Geometry: final body of the model. Coordinates: model frame, mm. A direction names the side the tool comes from. Coordinates: 2 decimals unless noted, no trailing zeros. Order: outer loops, then holes, each group sorted by start corner. A loop starts at its lowest first (then second) coordinate and runs counter-clockwise, first axis right, second up. Notation, with made-up numbers: (-30, 22.25) -> (20, 22.25) arc R9 ccw to (20, 27.25) -> close; hole circle Ø8 at (88, -23.5). An arc over 180 degrees is marked (long way). Answer in a Markdown table with one row per item. Add a question column.
1) Contact query for flat-ended pins moving along their axis: P1, Ø0.8, axis at y = 6.5, z = 29.5, coming from the +X side; P2, Ø0.6, axis at x = 14.5, z = 29.5, coming from the -Y side; P3, Ø1, axis at x = 14, z = 4.5, coming from the +Y side. Output: stop coordinate, or through.
2) Section query A-A on y = 9.5. Return the cut outline in (x, z), then the cut area to 4 significant figures.
3) Ray query, line 1 (Y direction, x = 4.5, z = 3); line 2 (X direction, y = 2.5, z = 20.5); line 3 (Z direction, x = 10.25, y = 13). Return the intervals inside material, ascending. Write a range as from..to.
4) Set-up query: faces 5 (the face through (14, 8, 1.5)), 6 (the face through (-0.5, 8, 29)), 7 (the face through (7, 16, 15)). Return all of +Z, -Z, +X, -X, +Y, -Y with unobstructed straight access to the full face (end or side cutting, diameter ignored); none if empty.
5) Pull-direction query (Y, two-part tool) for faces 1 (the face through (7, -1.3, 13)), 2 (the face through (7, 0, 15)), 3 (the face through (7, 27, -4)), 4 (the face through (14.5, 8, 7)); classes: +Y half, -Y half, draft (parallel to the pull), parting line (faces both ways), or undercut.
6) Section query C-C on x = 5. Return the cut outline in (y, z).
7) Section query B-B on z = -1.5. Return the cut outline in (x, y), then the cut area to 3 significant figures.
8) Section query D-D on z = 10. Return the cut outline in (x, y).
Autodesk Inventor part; units mm, degrees
ref_plane "Work Plane1" through (6.6, -1.3, -3) normal (1, 0, 0) x (0, 0, -1)
ref_plane "YZ Plane" through (0, 0, 0) normal (1, 0, 0) x (0, 1, 0)
ref_plane "XZ Plane" through (0, 0, 0) normal (0, 1, 0) x (-1, 0, 0)
sketch "Sketch1" plane through (0, 0, 0) normal (0, 0, 1) x (1, 0, 0)
  point P0 (0, 0)
sketch "Sketch2" plane through (0, 0, 0) normal (0, 0, 1) x (1, 0, 0)
  line L0 (0, 0) -> (13.2, 0)
  line L1 (13.2, 0) -> (13.2, 16)
  line L2 (13.2, 16) -> (0, 16)
  line L3 (0, 16) -> (0, 0)
  line L4 (14.5, 17.3) -> (14.5, -1.3)
  line L5 (14.5, -1.3) -> (-1.3, -1.3)
  line L6 (-1.3, -1.3) -> (-1.3, 17.3)
  line L7 (-1.3, 17.3) -> (14.5, 17.3)
  dimension "d0" = 13.2
  dimension "d1" = 16
  dimension "d2" = 1.3
extrude "Extrusion1" add sketch "Sketch2" along normal blind 30
sketch "Sketch3" plane through (0, 0, 0) normal (0, 0, -1) x (-1, 0, 0)
  line L0 (-14.5, -1.3) -> (-14.5, 17.3)
  line L1 (1.3, 17.3) -> (1.3, -1.3)
  line L2 (-14.5, 17.3) -> (1.3, 17.3)
  line L3 (1.3, -1.3) -> (-14.5, -1.3)
  line L4 (1.3, 17.3) -> (-14.5, 17.3)
  line L5 (-14.5, 17.3) -> (-14.5, 25.3)
  line L6 (-14.5, 25.3) -> (1.3, 25.3)
  line L7 (1.3, 25.3) -> (1.3, 17.3)
  line L8 (1.3, -1.3) -> (-14.5, -1.3)
  line L9 (-14.5, -1.3) -> (-14.5, -9.3)
  line L10 (-14.5, -9.3) -> (1.3, -9.3)
  line L11 (1.3, -9.3) -> (1.3, -1.3)
  point P0 (0, 0)
  dimension "d27" = 8
  dimension "d28" = 8
extrude "Extrusion2" add sketch "Sketch3" along normal blind 3 contours L0 L2 L1 L3
sketch "Sketch5" plane through (14.5, -1.3, 30) normal (1, 0, 0) x (0, 0, -1)
  line L0 (28.5, 2.8) -> (23.5, 2.8)
  line L1 (23.5, 2.8) -> (23.5, 15.8)
  line L2 (23.5, 15.8) -> (28.5, 15.8)
  line L3 (28.5, 15.8) -> (28.5, 2.8)
  line L4 (33, 0) -> (0, 0)
  line L5 (33, 18.6) -> (33, 0)
  point P0 (30, 1.3)
  point P1 (30, 0)
  dimension "d14" = 13
  dimension "d15" = 5
  dimension "d16" = 2.8
  dimension "d17" = 4.5
extrude "Extrusion4" cut sketch "Sketch5" against normal blind 1.3
sketch "Sketch6" plane through (-1.3, -1.3, 30) normal (-1, 0, 0) x (0, 0, 1)
  line L0 (0, 17.3) -> (0, 1.3)
  line L1 (0, 14.3) -> (-1.5, 14.3)
  line L2 (-1.5, 14.3) -> (-1.5, 4.3)
  line L3 (-1.5, 4.3) -> (0, 4.3)
  line L4 (0, 4.3) -> (0, 14.3)
  line L5 (0, 18.6) -> (-33, 18.6)
  point P0 (-30, 1.3)
  point P1 (0, 4.3)
  dimension "d20" = 10
  dimension "d21" = 1.5
  dimension "d30" = 4.3
sketch "Sketch7" plane through (14.5, -1.3, 30) normal (1, 0, 0) x (0, 0, -1)
  line L0 (1.5, 14.3) -> (1.5, 4.3)
  line L1 (0, 14.3) -> (1.5, 14.3)
  line L2 (1.5, 4.3) -> (0, 4.3)
  line L3 (0, 14.3) -> (0, 4.3)
  line L4 (0, 18.6) -> (0, 0)
  point P0 (30, 1.3)
  point P1 (0, 14.3)
ref_plane "Work Plane1" through (6.6, -1.3, -3) normal (1, 0, 0) x (0, 0, -1)
extrude "Extrusion7" cut sketch "Sketch7" against normal blind 0.8
extrude "Extrusion8" cut sketch "Sketch6" against normal blind 0.8
sketch "Sketch8" plane through (0, 0, -3) normal (0, 0, -1) x (-1, 0, 0)
  line L0 (-14.5, 28) -> (1.3, 28)
  line L1 (1.3, 28) -> (1.3, -12)
  line L2 (1.3, -12) -> (-14.5, -12)
  line L3 (-14.5, -12) -> (-14.5, 28)
  line L4 (1.3, 17.3) -> (-14.5, 17.3)
  line L5 (-14.5, -1.3) -> (1.3, -1.3)
  line L6 (-14.5, 17.3) -> (1.3, 17.3)
  line L7 (-14.5, 17.3) -> (-14.5, -1.3)
  line L8 (1.3, -1.3) -> (1.3, 17.3)
  line L9 (-14.5, 8) -> (1.3, 8) construction
  point P0 (0, 0)
  dimension "d39" = 40
  dimension "d40" = 20
extrude "Extrusion9" add sketch "Sketch8" along normal blind 5
fillet "Fillet2" radius 2 4 edges at (14.5, 17.3, 13.5) (-1.3, 17.3, 13.5) (14.5, -1.3, 13.5) (-1.3, -1.3, 13.5)
chamfer "Chamfer1" distance 2 angle 45 6 edges at (-1.3, 16.3, -3) (14.5, 16.3, -3) (-1.3, -0.3, -3) (14.5, -0.3, -3) (6.6, -12, -3) (6.6, 28, -3)
properties part number "VL53L0X_case"
Result:
| question | item | result |
|---|---|---|
| 1 | P1 | x = 13.7 |
| 1 | P2 | y = -0.35 |
| 1 | P3 | y = 17.03 |
| 2 | outline | (-1.3, -8) -> (14.5, -8) -> (14.5, 1.5) -> (13.2, 1.5) -> (13.2, 0) -> (0, 0) -> (0, 30) -> (-0.5, 30) -> (-0.5, 28.5) -> (-1.3, 28.5) -> close; (13.2, 6.5) -> (14.5, 6.5) -> (14.5, 28.5) -> (13.7, 28.5) -> (13.7, 30) -> (13.2, 30) -> close |
| 2 | area | 195.5 mm2 |
| 3 | line 1 | -1.3..0, 16..17.3 |
| 3 | line 2 | -1.3..0, 13.2..14.5 |
| 3 | line 3 | -8..0 |
| 4 | face 5 | +X |
| 4 | face 6 | +Z, -X |
| 4 | face 7 | +Z |
| 5 | face 1 | -Y half |
| 5 | face 2 | undercut |
| 5 | face 3 | +Y half |
| 5 | face 4 | draft |
| 6 | outline | (-12, -8) -> (28, -8) -> (28, -5) -> (26, -3) -> (17.3, -3) -> (17.3, 30) -> (16, 30) -> (16, 0) -> (0, 0) -> (0, 30) -> (-1.3, 30) -> (-1.3, -3) -> (-10, -3) -> (-12, -5) -> close |
| 7 | outline | (-1.3, 0.7) arc R2 ccw to (0.7, -1.3) -> (12.5, -1.3) arc R2 ccw to (14.5, 0.7) -> (14.5, 15.3) arc R2 ccw to (12.5, 17.3) -> (0.7, 17.3) arc R2 ccw to (-1.3, 15.3) -> close |
| 7 | area | 290 mm2 |
| 8 | outline | (-1.3, 0.7) arc R2 ccw to (0.7, -1.3) -> (12.5, -1.3) arc R2 ccw to (14.5, 0.7) -> (14.5, 15.3) arc R2 ccw to (12.5, 17.3) -> (0.7, 17.3) arc R2 ccw to (-1.3, 15.3) -> close; hole (0, 0) -> (13.2, 0) -> (13.2, 16) -> (0, 16) -> close |
